```python
from build123d import *

# Parameters (mm, degrees)
T_LE_DE_BASE_PLI_E1_DEPTH             = 20.5
ESQUISSE8_W                           = 24
ESQUISSE8_H                           = 2
BOSS_EXTRU_1_DEPTH                    = 8.5
T_LE_PLI_E_SUR_AR_TE1_STRIP_W         = 10
T_LE_PLI_E_SUR_AR_TE1_STRIP_H         = 2
T_LE_PLI_E_SUR_AR_TE1_STRIP_CUT_DEPTH = 8.5
T_LE_PLI_E_SUR_AR_TE1_DEPTH           = 8.5
ESQUISSE12_W                          = 1.5
ESQUISSE12_H                          = 12
ENL_V_MAT_EXTRU_1_DEPTH               = 8.5
DIAM_TRE_DU_PER_AGE_4_0_4_1_D         = 4
DIAM_TRE_DU_PER_AGE_8_0_8_1_D         = 8
DIAM_TRE_DU_PER_AGE_2_5_2_5_1_D       = 2.5
R_P_TITION_CIRCULAIRE1_COUNT          = 8
DIAM_TRE_DU_PER_AGE_4_0_4_2_D         = 4
HOLE_WIZARD_3_2_3_2_1_D               = 3.2
CONG_1_R                              = 4
DIAM_TRE_DU_PER_AGE_8_0_8_2_D         = 8
DIAM_TRE_DU_PER_AGE_2_5_2_5_3_D       = 2.5
R_P_TITION_CIRCULAIRE2_COUNT          = 4


# Sheet-metal steps are written as plain solids
with BuildPart() as part:
    # Esquisse1 → Tôle de base pliée1 (new body)
    with BuildSketch(Plane(origin=(0, 0, 0), x_dir=(0, 0, -1), z_dir=(1, 0, 0))):
        with BuildLine():
            Line((0, 27), (0, 3))
            ThreePointArc((0, 3), (-0.878679656, 0.878679656), (-3, 0))
            Line((-3, 0), (-37.5, 0))
            Line((-37.5, 0), (-37.5, 2))
            Line((-37.5, 2), (-3, 2))
            ThreePointArc((-3, 2), (-2.292893219, 2.292893219), (-2, 3))
            Line((-2, 3), (-2, 27))
            Line((-2, 27), (0, 27))
        make_face()
    extrude(amount=T_LE_DE_BASE_PLI_E1_DEPTH)

    # Esquisse8 → Boss.-Extru.1 (add)
    with BuildSketch(Plane(origin=(20.5, 0, 0), x_dir=(0, 0, -1), z_dir=(1, 0, 0))):
        with Locations((-19, 1)):
            Rectangle(ESQUISSE8_W, ESQUISSE8_H)
    extrude(amount=BOSS_EXTRU_1_DEPTH)

    # Tôle pliée sur arête1 strip (across the edge) → Tôle pliée sur arête1 strip cut (cut)
    with BuildSketch(Plane(origin=(20.5, 2, 31), x_dir=(0, 0, -1), z_dir=(1, 0, 0))):
        with Locations((-4, -1)):
            Rectangle(T_LE_PLI_E_SUR_AR_TE1_STRIP_W, T_LE_PLI_E_SUR_AR_TE1_STRIP_H)
    extrude(amount=T_LE_PLI_E_SUR_AR_TE1_STRIP_CUT_DEPTH, mode=Mode.SUBTRACT)

    # Tôle pliée sur arête1 section (across the edge) → Tôle pliée sur arête1 (add)
    with BuildSketch(Plane(origin=(20.5, 2, 31), x_dir=(0, 0, -1), z_dir=(1, 0, 0))):
        with BuildLine():
            Line((-2, 1), (-2, 25))
            Line((-2, 25), (0, 25))
            Line((0, 25), (0, 1))
            ThreePointArc((0, 1), (0.292893219, 0.292893219), (1, 0))
            Line((1, 0), (1, -2))
            ThreePointArc((1, -2), (-1.121320344, -1.121320344), (-2, 1))
        make_face()
    extrude(amount=T_LE_PLI_E_SUR_AR_TE1_DEPTH)

    # Esquisse12 → Enlèv. mat.-Extru.1 (cut)
    with BuildSketch(Plane(origin=(0, 2, 0), x_dir=(1, 0, 0), z_dir=(0, 1, 0))):
        with Locations((19.75, -31.5)):
            Rectangle(ESQUISSE12_W, ESQUISSE12_H)
    extrude(amount=-ENL_V_MAT_EXTRU_1_DEPTH, mode=Mode.SUBTRACT)

    # Diamètre du perçage Ø4.0 (4)1 (through all)
    with Locations(Plane(origin=(0, 2, 0), x_dir=(1, 0, 0), z_dir=(0, 1, 0))):
        with Locations((24.25, -12.13), (24.25, -22.13)):
            Hole(DIAM_TRE_DU_PER_AGE_4_0_4_1_D / 2)

    # Diamètre du perçage Ø8.0 (8)1 (through all)
    with Locations(Plane(origin=(0, 2, 0), x_dir=(1, 0, 0), z_dir=(0, 1, 0))):
        with Locations((9.75, -25.5)):
            Hole(DIAM_TRE_DU_PER_AGE_8_0_8_1_D / 2)

    # Diamètre du perçage Ø2.5 (2.5)1 (through all)
    with Locations(Plane(origin=(0, 2, 0), x_dir=(1, 0, 0), z_dir=(0, 1, 0))):
        with Locations((9.75, -18.5)):
            diam_tre_du_per_age_2_5_2_5_1 = Hole(DIAM_TRE_DU_PER_AGE_2_5_2_5_1_D / 2)

    # Répétition circulaire1: Diamètre du perçage Ø2.5 (2.5)1 ×8 about axis, 3 skipped
    r_p_tition_circulaire1_axis = Axis((9.75, 2, 25.5), (0, 1, 0))
    add([diam_tre_du_per_age_2_5_2_5_1.rotate(r_p_tition_circulaire1_axis, i * 360 / R_P_TITION_CIRCULAIRE1_COUNT) for i in range(1, R_P_TITION_CIRCULAIRE1_COUNT) if i not in (1, 3, 6)], mode=Mode.SUBTRACT)

    # Diamètre du perçage Ø4.0 (4)2 (through all)
    with Locations(Plane.XY.offset(33)):
        with Locations((24.25, 19.87), (24.25, 9.87)):
            Hole(DIAM_TRE_DU_PER_AGE_4_0_4_2_D / 2)

    # Ø3.2 (3.2) 直径孔1 (through all)
    with Locations(Plane.XY.offset(2)):
        with Locations((10.5, 14.87), (10.5, 21.87), (17.5, 14.87), (10.5, 7.87), (3.5, 14.87)):
            Hole(HOLE_WIZARD_3_2_3_2_1_D / 2)

    # Congé1
    cong_1_edges = [part.edges().sort_by_distance(p)[0] for p in [
        (20.5, 27, 1),
        (29, 1, 7),
        (29, 27, 32),
        (19, 1, 37.5),
    ]]
    fillet(cong_1_edges, radius=CONG_1_R)

    # Symétrie1: part across plane


with BuildPart() as part_1:
    add(part.part)
    add(part.part.mirror(Plane(origin=(0, 3, 3), x_dir=(0, 0, 1), z_dir=(1, 0, 0))))

    # Diamètre du perçage Ø8.0 (8)2 (through all)
    with Locations(Plane(origin=(0, 2, 0), x_dir=(1, 0, 0), z_dir=(0, 1, 0))):
        with Locations((0, -12.13)):
            Hole(DIAM_TRE_DU_PER_AGE_8_0_8_2_D / 2)

    # Diamètre du perçage Ø2.5 (2.5)3 (through all)
    with Locations(Plane(origin=(0, 2, 0), x_dir=(1, 0, 0), z_dir=(0, 1, 0))):
        with Locations((0, -5.13)):
            diam_tre_du_per_age_2_5_2_5_3 = Hole(DIAM_TRE_DU_PER_AGE_2_5_2_5_3_D / 2)

    # Répétition circulaire2: Diamètre du perçage Ø2.5 (2.5)3 ×4 about axis
    r_p_tition_circulaire2_axis = Axis((0, 0, 12.13), (0, 1, 0))
    for i in range(1, R_P_TITION_CIRCULAIRE2_COUNT):
        add(diam_tre_du_per_age_2_5_2_5_3.rotate(r_p_tition_circulaire2_axis, i * 360 / R_P_TITION_CIRCULAIRE2_COUNT), mode=Mode.SUBTRACT)


solid = part_1.part
```
The listing builds one solid part. Answer for the finished solid, in the listing's coordinates (mm). A direction names the side the tool comes from. Give positions to 0.01 mm unless a question says otherwise; leave off trailing zeros. Order: outer loops, then holes, each group sorted by start corner. A loop starts at its lowest first (then second) coordinate and runs counter-clockwise, first axis right, second up. Notation, with made-up numbers: (24, 16) -> (47, 16) arc R13 ccw to (47, 23) -> close; hole circle Ø5 at (23, -23). An arc over 180 degrees is marked (long way). Answer as a JSON object with one key per item and string values. Group by question number.
Item 1: Determine the mould class of faces 1 (the cylindrical face through (-11.68, 22.95, 0.99)), 2 (the cylindrical face through (-8.5, 0.99, 32.55)), 3 (the flat face through (0, 27, 1)) for opening direction Y: pulls with the +Y half, pulls with the -Y half, needs draft (parallel to the pull), parting line crosses it, or undercut.
Item 2: Flat-ended cylindrical pins translate along their axes: pin 1 (4.5 mm diameter, centred on x = -24.25, y = 9.87, fed in from +Z); pin 2 (8 mm diameter, centred on x = -3.5, y = 20.5, fed in from +Z); pin 3 (4 mm diameter, centred on x = 17, z = 16, fed in from +Y). Find the tip coordinate at first contact, or state that the pin passes through.
Item 3: The part is cut by section C-C on x = 17.5. Write down the section's boundary in (y, z).
Item 4: The part is cut by section B-B on z = 12.13. Write down the section's boundary in (x, y), and give its area (3 significant figures).
Item 5: The part is cut by section A-A on z = 5.13. Write down the section's boundary in (x, y), and give its area (3 significant figures).
Item 6: The part is cut by section D-D on y = 19. Write down the section's boundary in (x, z).
Item 7: Consider L1, parallel to Y at x = 24.25, z = 32.3; L2, parallel to Z at x = -24.25, y = 1.5; L3, parallel to Z at x = 15, y = 23.5. Determine where each line is inside the solid, lowest interval first. Write a range as from..to.
Item 8: A tool of negligible diameter and unlimited length cuts with its end or side. For faces 4 (the flat face through (25, 15, 31)), 5 (the cylindrical face through (25.837, 0.986, 13.347)), 6 (the flat face through (20.5, 12, 32)), from which of +Z, -Z, +X, -X, +Y, -Y can it reach the whole face along a straight path? Write none if from no direction.
Result set:
{
 "1": {"face 1": "undercut", "face 2": "needs draft", "face 3": "pulls with the +Y half"},
 "2": {"pin 1": "z = 33", "pin 2": "z = 2", "pin 3": "y = 2"},
 "3": {"outline": "(0, 3) arc R3 ccw to (3, 0) -> (13.27, 0) -> (13.27, 2) -> (3, 2) arc R1 cw to (2, 3) -> (2, 36.62) -> (0, 36.62) -> close; (16.47, 0) -> (26.87, 0) -> (26.87, 2) -> (16.47, 2) -> close"},
 "4": {"outline": "(-29, 0) -> (-26.25, 0) -> (-26.25, 2) -> (-29, 2) -> close; (-22.25, 0) -> (-8.25, 0) -> (-8.25, 2) -> (-22.25, 2) -> close; (-5.75, 0) -> (-4, 0) -> (-4, 2) -> (-5.75, 2) -> close; (4, 0) -> (5.75, 0) -> (5.75, 2) -> (4, 2) -> close; (8.25, 0) -> (22.25, 0) -> (22.25, 2) -> (8.25, 2) -> close; (26.25, 0) -> (29, 0) -> (29, 2) -> (26.25, 2) -> close", "area": "74.0 mm²"},
 "5": {"outline": "(-20.5, 0) -> (-1.25, 0) -> (-1.25, 2) -> (-20.5, 2) -> close; (1.25, 0) -> (20.5, 0) -> (20.5, 2) -> (1.25, 2) -> close", "area": "77.0 mm²"},
 "6": {"outline": "(-29, 31) -> (-26.05, 31) -> (-26.05, 33) -> (-29, 33) -> close; (-22.45, 31) -> (-20.5, 31) -> (-20.5, 33) -> (-22.45, 33) -> close; (-20.5, 0) -> (20.5, 0) -> (20.5, 2) -> (-20.5, 2) -> close; (20.5, 31) -> (22.45, 31) -> (22.45, 33) -> (20.5, 33) -> close; (26.05, 31) -> (29, 31) -> (29, 33) -> (26.05, 33) -> close"},
 "7": {"L1": "1.07..7.87, 11.87..17.87, 21.87..27", "L2": "7..10.13, 14.13..20.13, 24.13..32.6", "L3": "0..2"},
 "8": {"face 4": "-Z, +X, -X, +Y", "face 5": "+Y, -Y", "face 6": "+Z, +Y, -Y"}
}
